from build123d import *

# Parameters (mm, degrees)
BOSS_EXTRUDE1_DEPTH     = 101.6
CUT_EXTRUDE1_DEPTH      = 165.61081374
CUT_EXTRUDE1_DEPTH_BACK = 165.61081374
FILLET6_R               = 6.35
FILLET7_R               = 6.35


with BuildPart() as part:
    # Sketch1 → Boss-Extrude1 (new body)
    with BuildSketch(Plane.XY):
        with BuildLine():
            Line((0, 0), (25.4, 0))
            Line((25.4, 0), (25.4, 114.3))
            ThreePointArc((25.4, 114.3), (12.7, 127), (0, 114.3))
            Line((0, 114.3), (0, 0))
        make_face()
    extrude(amount=BOSS_EXTRUDE1_DEPTH)

    # Sketch2 → Cut-Extrude1 (cut, two sides: drawn at the far end of the back side and taken through both)
    with BuildSketch(Plane(origin=(25.4, 0, 0), x_dir=(0, 0, -1), z_dir=(1, 0, 0)).offset(-CUT_EXTRUDE1_DEPTH_BACK)):
        with BuildLine():
            Line((-76.2, 107.95), (-25.4, 107.95))
            ThreePointArc((-25.4, 107.95), (-12.7, 95.25), (-25.4, 82.55))
            Line((-25.4, 82.55), (-76.2, 82.55))
            ThreePointArc((-76.2, 82.55), (-88.9, 95.25), (-76.2, 107.95))
        make_face()
    extrude(amount=CUT_EXTRUDE1_DEPTH + CUT_EXTRUDE1_DEPTH_BACK, mode=Mode.SUBTRACT)

    # Fillet6
    fillet6_edges = [part.edges().sort_by_distance(p)[0] for p in [
        (0, 95.25, 88.9),
        (0, 95.25, 12.7),
        (0, 82.55, 50.8),
        (0, 107.95, 50.8),
    ]]
    fillet(fillet6_edges, radius=FILLET6_R - 0.0001)  # a hair under: the kernel refuses the full size

    # Fillet7
    fillet7_edges = [part.edges().sort_by_distance(p)[0] for p in [
        (25.4, 82.55, 50.8),
        (25.4, 95.25, 12.7),
        (25.4, 107.95, 50.8),
        (25.4, 95.25, 88.9),
    ]]
    fillet(fillet7_edges, radius=FILLET7_R - 0.0001)  # a hair under: the kernel refuses the full size


solid = part.part
CAD build for the part. Positions are in the model's coordinates, mm. A direction names the side the tool comes from. Round coordinates to 2 decimals unless told otherwise and drop trailing zeros. Write each loop counter-clockwise with the first axis right and the second up, starting at its lowest first coordinate (ties: lowest second). Pieces come first, ordered by that corner, then holes.
(1) Slice it at C-C, the plane y = 95.25. Write the cut outline in (x, z).
(2) Slice it at D-D, the plane x = 21.5. Write the cut outline in (y, z).
(3) Probe line 1 along Y through (x, z) = (5.25, 24); line 2 along Y through (x, z) = (13, 25); line 3 along Z through (x, y) = (23.25, 98). List the from-to ranges inside material, lowest first.
(4) Slice it at B-B, the plane x = 12.7. Write the cut outline in (y, z).
(5) 3-axis set-ups, long thin cutter, end or side, ignore diameter. For faces 1 (the face through (1.81, 109.86, 50.44)), 2 (the face through (12.611, 94.971, 88.897)), 3 (the face through (13, 64, 101.6)), 4 (the face through (23.49, 109.76, 50.44)): which of +Z, -Z, +X, -X, +Y, -Y reach the whole face in a straight line?
(6) Drop a flat-ended pin along its axis: P1, Ø1.5, axis at x = 21, z = 72.5, coming from the +Y side. Give the stop position or say it passes through.
From the geometry:
1. outline: (0, 0) - (25.4, 0) - (25.4, 6.35) arc R6.35 ccw to (19.05, 12.7) - (6.35, 12.7) arc R6.35 ccw to (0, 6.35) - close; (0, 95.25) arc R6.35 ccw to (6.35, 88.9) - (19.05, 88.9) arc R6.35 ccw to (25.4, 95.25) - (25.4, 101.6) - (0, 101.6) - close
2. outline: (0, 0) - (123.46, 0) - (123.46, 101.6) - (0, 101.6) - close; hole (82.06, 25.4) arc R13.19 ccw to (108.44, 25.4) - (108.44, 76.2) arc R13.19 ccw to (82.06, 76.2) - close
3. line 1: y = 0 to 82.53, 107.97 to 124.59
3. line 2: y = 0 to 82.56, 107.94 to 127
3. line 3: z = 0 to 11.38, 90.22 to 101.6
4. outline: (0, 0) - (127, 0) - (127, 101.6) - (0, 101.6) - close; hole (82.55, 25.4) arc R12.7 ccw to (107.95, 25.4) - (107.95, 76.2) arc R12.7 ccw to (82.55, 76.2) - close
5. face 1: -X
5. face 2: +X, -X
5. face 3: +Z, +X, -X, +Y, -Y
5. face 4: +X
6. P1: stops at y = 124.51
